from build123d import *

# Parameters (mm, degrees)
F0_W      = 38.1
F0_H      = 38.1
F1_DEPTH  = 38.1
F5_W      = 25.4
F5_H      = 7.62
F6_DEPTH  = 38.1
F8_DEPTH  = 38.1
F10_DEPTH = 38.1


with BuildPart() as f1:
    # F0 (on Front) → F1 (new body)
    with BuildSketch(Plane.XZ):
        with Locations((19.05, 19.05)):
            Rectangle(F0_W, F0_H)
    extrude(amount=F1_DEPTH)

    # F5 (on offset) → F6 (cut)
    with BuildSketch(Plane.YZ.offset(38.1)):
        with Locations((-12.7, 26.67)):
            Rectangle(F5_W, F5_H)
        with Locations((-25.4, 11.43)):
            Rectangle(F5_W, F5_H)
    extrude(amount=-F6_DEPTH, mode=Mode.SUBTRACT)

    # F7 (on offset) → F8 (cut)
    with BuildSketch(Plane.XZ.offset(38.1)):
        Polygon((0, 38.1), (0, 0), (12.7, 38.1), align=None)
        Polygon((19.05, 17.435988), (12.7, 0), (25.4, 0), align=None)
        Polygon((23.515154, 22.983656), (19.499061, 35.031934), (15.482969, 22.983656), align=None)
        Polygon((38.1, 38.1), (25.4, 38.1), (38.1, 0), align=None)
    extrude(amount=-F8_DEPTH, mode=Mode.SUBTRACT)

    # F9 (on offset) → F10 (cut)
    with BuildSketch(Plane.XY.offset(38.1)):
        Polygon((6.35, 0), (0, 0), (0, -38.1), align=None)
        Polygon((11.43, -15.875), (6.35, -38.1), (31.75, -38.1), (26.67, -15.875), (21.59, -28.575), (16.51, -28.575), align=None)
        Polygon((25.4, 0), (12.7, 0), (19.05, -15.875), align=None)
        Polygon((38.1, 0), (31.75, 0), (38.1, -38.1), align=None)
    extrude(amount=-F10_DEPTH, mode=Mode.SUBTRACT)


solid = f1.part
Input: part model. Units: mm. Frame: model coordinates. A direction names the side the tool comes from. Coordinates: 2 decimals unless noted, no trailing zeros. Loops run counter-clockwise (first coordinate to the right, second up) from the corner with the lowest first, then second, coordinate; pieces in that order, holes last. Notation, with made-up numbers: (-16.5, 17) -> (24.5, 17) arc R25 cw to (24.5, 44) -> close; hole circle Ø9 at (65.5, 11). An arc over 180 degrees is marked (long way). One line per item, written item: value.
(1) Cut plane D-D (y = -17). Give the number of separate pieces and of enclosed holes in the cut face, then the cut area to 3 significant figures.
Answer below:
separate pieces: 10
enclosed holes: 0
area: 435 mm2
(2) Draft query along Z for faces 4 (the face through (10, -20, 15.24)), 5 (the face through (19, -17, 38.1)), 6 (the face through (20.456, -21.848, 32.161)), 7 (the face through (29.246, -27.143, 3.863)). Return one class per face: pulls with the +Z half, pulls with the -Z half, needs draft (parallel to the pull), parting line crosses it, or undercut.
Answer below:
face 4: undercut
face 5: pulls with the +Z half
face 6: undercut
face 7: needs draft
(3) Cut plane A-A (z = 4.5). Output: boundary loops of the cut face in (x, y) (3 decimals), then the cut area to 3 significant figures.
Answer below:
outline: (1.5, -38.1) -> (6.35, -38.1) -> (11.43, -15.875) -> (14.339, -23.147) -> (14.339, -4.097) -> (12.7, 0) -> (6.35, 0) -> (1.5, -29.1) -> close; (23.761, -23.147) -> (26.67, -15.875) -> (31.75, -38.1) -> (36.6, -38.1) -> (36.6, -29.1) -> (31.75, 0) -> (25.4, 0) -> (23.761, -4.097) -> close
area: 609 mm2
(4) Ray query, line 1 along Z through (x, y) = (17, -17); line 2 along Z through (x, y) = (9, -2.5); line 3 along X through (y, z) = (-10.5, 32). Return the intervals inside material, ascending.
Answer below:
line 1: z = 15.24 to 22.86, 30.48 to 38.1
line 2: z = 0 to 22.86
line 3: x = 10.67 to 16.9, 21.2 to 27.43
(5) Cut plane C-C (x = 35). Output: boundary loops of the cut face in (y, z).
Answer below:
outline: (-38.1, 0) -> (-19.5, 0) -> (-19.5, 7.62) -> (-38.1, 7.62) -> close
(6) Set-up query: faces 1 (the face through (29.246, -27.143, 18.805)), 2 (the face through (4, -38.1, 4)), 3 (the face through (16.5, -25.4, 26.9)). Return all of +Z, -Z, +X, -X, +Y, -Y with unobstructed straight access to the full face (end or side cutting, diameter ignored); none if empty.
Answer below:
face 1: +Z, -Z, -Y
face 2: +Z, -Z, +X, -X, -Y
face 3: +X, -X, +Y
(7) Cut plane B-B (z = 24). Output: boundary loops of the cut face in (x, y).
Answer below:
outline: (8, -30.88) -> (9.25, -25.4) -> (8, -25.4) -> close; (15.24, -25.4) -> (15.82, -26.85) -> (15.82, -25.4) -> close; (28.85, -25.4) -> (30.1, -30.88) -> (30.1, -25.4) -> close
(8) Pin query (flat end, axial travel): pin 1 Ø0.5 at (x, z) = (29.5, 26) entering from +Y; pin 2 Ø5 at (y, z) = (-5, 33.5) entering from -X; pin 3 Ø6 at (x, z) = (29.5, 11.5) entering from +Y; pin 4 Ø4 at (x, z) = (18, 32.5) entering from -Y (3 decimals). Return the tip coordinate at first contact, or that it passes through.
Answer below:
pin 1: stops at y = -25.4
pin 2: stops at x = 10.33
pin 3: stops at y = 0
pin 4: stops at y = -28.575
